```python
from build123d import *

# Parameters (mm, degrees)
F0_W       = 36
F0_H       = 15
F1_DEPTH   = 7
F2_W       = 36
F2_H       = 2.5
F3_DEPTH   = 30
F3_FACE1_W = 36
F3_FACE1_H = 30
F5_DEPTH   = 25
F6_D       = 5.1054


with BuildPart() as f1:
    # F0 (on Top) → F1 (new body)
    with BuildSketch(Plane.XY):
        Rectangle(F0_W, F0_H)
    extrude(amount=F1_DEPTH)

    # F2 (on face) → F3 (join)
    with BuildSketch(Plane.XY.offset(7)):
        with Locations((0, 6.25)):
            Rectangle(F2_W, F2_H)
    extrude(amount=F3_DEPTH)

    # F4 (on face) + F3_face1 (on face) → F5 (cut)
    with BuildSketch(Plane(origin=(0, 7.5, 0), x_dir=(-1, 0, 0), z_dir=(0, 1, 0))):
        with BuildLine():
            Line((-18, 37), (-18, 28.4477328312))
            ThreePointArc((-18, 28.4477328312), (0, 24.7), (18, 28.4477328312))
            Line((18, 28.4477328312), (18, 37))
            Line((18, 37), (-18, 37))
        make_face()
    with BuildSketch(Plane(origin=(0, 5, 22), x_dir=(1, 0, 0), z_dir=(0, -1, 0))):
        Rectangle(F3_FACE1_W, F3_FACE1_H)
    extrude(amount=-F5_DEPTH, dir=(0, 1, 0), mode=Mode.SUBTRACT)

    # F6 (through all)
    with Locations(Plane(origin=(0, 0, 0), x_dir=(1, 0, 0), z_dir=(0, 0, -1))):
        with Locations((0, 0)):
            Hole(F6_D / 2)


solid = f1.part
```
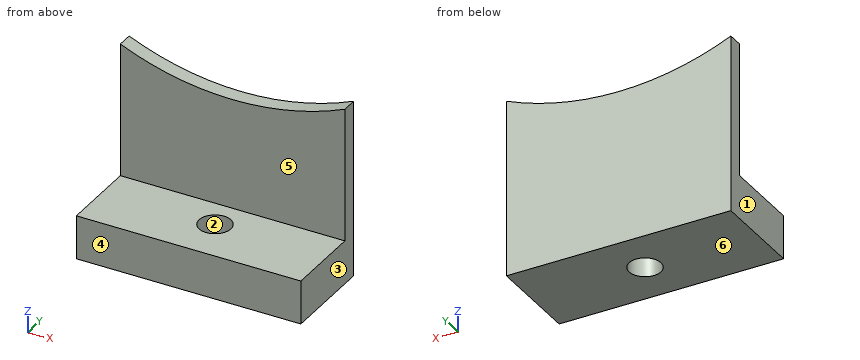
Can you work these out from the model? Positions are in its coordinate system, mm. Face numbers are marked on the shaded views. A direction names the side the tool comes from. Round coordinates to 2 decimals unless told otherwise and drop trailing zeros. Loops run counter-clockwise (first coordinate to the right, second up) from the corner with the lowest first, then second, coordinate; pieces in that order, holes last. Notation, with made-up numbers: (25, -0.75) -> (47, -0.75) arc R24 ccw to (47, 26.25) -> close; hole circle Ø11 at (48, 23). An arc over 180 degrees is marked (long way). One line per item, written item: value. Start each with the question number.
1. If we section it at B-B, the plane y = 0: Write out the boundary of the cut face in (x, z).
2. If I drill on probe 1 along Y at (x, z) = (0, 4); probe 2 along Z at (x, y) = (14, -2.75); probe 3 along Y at (x, z) = (8, 23.5), over which ranges is the centre line in solid material (lowest first)?
3. If we mould it in two halves opening along X, with no side actions, what happens to the marked faces 1, 2, 3 and 4? For each: pulls with the +X half, pulls with the -X half, needs draft (parallel to the pull), parting line crosses it, or undercut.
4. For the marked faces 5 and 6, which set-ups out of +Z, -Z, +X, -X, +Y, -Y let a thin tool reach every point of the face, with its end or its side?
5. If we section it at A-A, the plane x = 0: Write out the boundary of the cut face in (y, z), then the cut area to 3 significant figures.
6. For pin 1 (1 mm diameter, centred on x = -14, z = 13, fed in from -Y); pin 2 (6 mm diameter, centred on x = 0, y = 0, fed in from +Z), each with a flat end and sliding along its axis, tell me the tip position at first contact or that it passes through.
7. If we section it at C-C, the plane y = 2: Write out the boundary of the cut face in (x, z), then the cut area to 3 significant figures.
8. If we section it at D-D, the plane x = -8.5: Write out the boundary of the cut face in (y, z).
Calculated:
1. outline: (-18, 0) -> (-2.55, 0) -> (-2.55, 7) -> (-18, 7) -> close; (2.55, 0) -> (18, 0) -> (18, 7) -> (2.55, 7) -> close
2. probe 1: y = -7.5 to -2.55, 2.55 to 7.5
2. probe 2: z = 0 to 7
2. probe 3: y = 5 to 7.5
3. face 1: pulls with the -X half
3. face 2: undercut
3. face 3: pulls with the +X half
3. face 4: needs draft
4. face 5: +Z, +X, -X, -Y
4. face 6: -Z, +X, -X, +Y, -Y
5. outline: (-7.5, 0) -> (-2.55, 0) -> (-2.55, 7) -> (-7.5, 7) -> close; (2.55, 0) -> (7.5, 0) -> (7.5, 24.7) -> (5, 24.7) -> (5, 7) -> (2.55, 7) -> close
5. area: 114 mm²
6. pin 1: stops at y = 5
6. pin 2: stops at z = 7
7. outline: (-18, 0) -> (-1.59, 0) -> (-1.59, 7) -> (-18, 7) -> close; (1.59, 0) -> (18, 0) -> (18, 7) -> (1.59, 7) -> close
7. area: 230 mm²
8. outline: (-7.5, 0) -> (7.5, 0) -> (7.5, 25.51) -> (5, 25.51) -> (5, 7) -> (-7.5, 7) -> close
